from build123d import *

# Parameters (mm, degrees)
SKETCH_1_R          = 10
EXTRUDE_1_DEPTH     = 1
SKETCH_2_R          = 27.5
EXTRUDE_2_DEPTH     = 3.5
SKETCH_3_R          = 8.5
EXTRUDE_3_DEPTH     = 33
SKETCH_4_R          = 5
CUT_EXTRUDE_1_DEPTH = 20
EXTRUDE_START       = -37.5
EXTRUDE_4_DEPTH     = 37.5
SKETCH_9_R          = 1.5
CUT_EXTRUDE_4_DEPTH = 15
SKETCH_10_R         = 9.5
SKETCH_10_R_2       = 8.5
EXTRUDE_5_DEPTH     = 9.3
FILLET_2_R          = 8
CHAMFER_1_SIZE      = 0.5
CHAMFER_2_SIZE      = 0.5
SKETCH_12_R         = 1.5
CUT_EXTRUDE_6_DEPTH = 20
SKETCH_13_R         = 3.75
CUT_EXTRUDE_7_DEPTH = 44.732139257
FILLET_3_R          = 1
CHAMFER_3_SIZE      = 0.5
SKETCH_14_R         = 2.6
CUT_EXTRUDE_8_DEPTH = 10


with BuildPart() as part:
    # 草图1 → 凸台-拉伸1 (new body)
    with BuildSketch(Plane(origin=(0, 0, 0), x_dir=(1, 0, 0), z_dir=(0, 1, 0))):
        with Locations(Location((0, 0, 0), (0, 0, 270))):
            Circle(SKETCH_1_R)
    extrude(amount=EXTRUDE_1_DEPTH)

    # 草图2 → 凸台-拉伸2 (add)
    with BuildSketch(Plane(origin=(0, 1, 0), x_dir=(1, 0, 0), z_dir=(0, 1, 0))):
        with Locations(Location((0, 0, 0), (0, 0, 270))):
            Circle(SKETCH_2_R)
    extrude(amount=EXTRUDE_2_DEPTH)

    # 草图3 → 凸台-拉伸3 (add)
    with BuildSketch(Plane(origin=(0, 4.5, 0), x_dir=(1, 0, 0), z_dir=(0, 1, 0))):
        with Locations(Location((0, 0, 0), (0, 0, 270))):
            Circle(SKETCH_3_R)
    extrude(amount=EXTRUDE_3_DEPTH)

    # 草图4 → 切除-拉伸1 (cut)
    with BuildSketch(Plane(origin=(0, 37.5, 0), x_dir=(1, 0, 0), z_dir=(0, 1, 0))):
        with Locations(Location((0, 0, 0), (0, 0, 270))):
            Circle(SKETCH_4_R)
    extrude(amount=-CUT_EXTRUDE_1_DEPTH, mode=Mode.SUBTRACT)

    # 草图8 → 凸台-拉伸4 (add)
    with BuildSketch(Plane.XZ.offset(EXTRUDE_START)):
        with BuildLine():
            Line((4, 3), (4, -3))
            ThreePointArc((4, -3), (5, 0), (4, 3))
        make_face()
    extrude(amount=EXTRUDE_4_DEPTH)

    # 草图9 → 切除-拉伸4 (cut, symmetric)
    with BuildSketch(Plane.ZY.offset(-4)):
        with Locations((0, 28.5)):
            Circle(SKETCH_9_R)
    extrude(amount=CUT_EXTRUDE_4_DEPTH, both=True, mode=Mode.SUBTRACT)

    # 草图10 → 凸台-拉伸5 (add)
    with BuildSketch(Plane(origin=(0, 4.5, 0), x_dir=(1, 0, 0), z_dir=(0, 1, 0))):
        with Locations(Location((0, 0, 0), (0, 0, 270))):
            Circle(SKETCH_10_R)
        with Locations(Location((0, 0, 0), (0, 0, 270))):
            Circle(SKETCH_10_R_2, mode=Mode.SUBTRACT)
    extrude(amount=EXTRUDE_5_DEPTH)

    # 圆角2
    fillet_2_edges = [part.edges().sort_by_distance(p)[0] for p in [
        (0, 4.5, -9.5),
    ]]
    fillet(fillet_2_edges, radius=FILLET_2_R)

    # 倒角1
    chamfer_1_edges = [part.edges().sort_by_distance(p)[0] for p in [
        (0, 4.5, -27.5),
    ]]
    chamfer(chamfer_1_edges, length=CHAMFER_1_SIZE)

    # 倒角2
    chamfer_2_edges = [part.edges().sort_by_distance(p)[0] for p in [
        (0, 37.5, -8.5),
    ]]
    chamfer(chamfer_2_edges, length=CHAMFER_2_SIZE)

    # 草图12 → 切除-拉伸6 (cut)
    with BuildSketch(Plane(origin=(0, 37.5, 0), x_dir=(1, 0, 0), z_dir=(0, 1, 0))):
        with Locations((3, 3.5)):
            Circle(SKETCH_12_R)
        with Locations((3, -3.5)):
            Circle(SKETCH_12_R)
    extrude(amount=-CUT_EXTRUDE_6_DEPTH, mode=Mode.SUBTRACT)

    # 草图13 → 切除-拉伸7 (cut, through all)
    with BuildSketch(Plane(origin=(0, 17.5, 0), x_dir=(1, 0, 0), z_dir=(0, 1, 0))):
        with Locations(Location((0, 0, 0), (0, 0, 270))):
            Circle(SKETCH_13_R)
    extrude(amount=-CUT_EXTRUDE_7_DEPTH, mode=Mode.SUBTRACT)

    # 圆角3
    fillet_3_edges = [part.edges().sort_by_distance(p)[0] for p in [
        (1.973716593, 27.5, -4.593957206),
        (1.973716593, 27.5, 4.593957206),
    ]]
    fillet(fillet_3_edges, radius=FILLET_3_R)

    # 倒角3
    chamfer_3_edges = [part.edges().sort_by_distance(p)[0] for p in [
        (0, 1, -27.5),
    ]]
    chamfer(chamfer_3_edges, length=CHAMFER_3_SIZE)

    # 草图14 → 切除-拉伸8 (cut)
    with BuildSketch(Plane.XZ.offset(-1)):
        with Locations(Location((22.5, 0, 0), (0, 0, 270))):
            Circle(SKETCH_14_R)
        with Locations(Location((11.25, -19.485571585, 0), (0, 0, 270))):
            Circle(SKETCH_14_R)
        with Locations(Location((-11.25, -19.485571585, 0), (0, 0, 270))):
            Circle(SKETCH_14_R)
        with Locations(Location((-22.5, 0, 0), (0, 0, 270))):
            Circle(SKETCH_14_R)
        with Locations(Location((-11.25, 19.485571585, 0), (0, 0, 270))):
            Circle(SKETCH_14_R)
        with Locations(Location((11.25, 19.485571585, 0), (0, 0, 270))):
            Circle(SKETCH_14_R)
    extrude(amount=-CUT_EXTRUDE_8_DEPTH, mode=Mode.SUBTRACT)


solid = part.part
Part model, mm, in its own coordinate system. A direction names the side the tool comes from. Coordinates: 2 decimals unless noted, no trailing zeros. Write each loop counter-clockwise with the first axis right and the second up, starting at its lowest first coordinate (ties: lowest second). Pieces come first, ordered by that corner, then holes. Notation, with made-up numbers: M -35.5,-26 L -14.5,-26 A13 ccw -14.5,-15 Z; hole C 6.5,84.25 d4. An arc over 180 degrees is marked long. Return JSON: item names as keys, results as strings.
1. 3-axis set-ups, long thin cutter, end or side, ignore diameter. For faces 4 (the face through (0, 1, 12)), 5 (the face through (-12.246, 2.726, 17.084)), 6 (the face through (-5.78, 13.14, -7.54)): which of +Z, -Z, +X, -X, +Y, -Y reach the whole face in a straight line?
Determined:
{"face 4": "-Y", "face 5": "+Y, -Y", "face 6": "+Y"}
2. Probe L1, parallel to Y at x = -10.5, z = -16; L2, parallel to X at y = 23, z = -7; L3, parallel to X at y = 20, z = 4.5. List the from-to ranges inside material, lowest first.
Determined:
{"L1": "1 to 4.5", "L2": "-4.82 to 4.82", "L3": "-7.21 to -2.18, 4.12 to 7.21"}
3. Flat gauge pins, fed straight in: pin 1 Ø8.5 at (x, z) = (11.25, 19.49) entering from -Y; pin 2 Ø12 at (x, z) = (-14.5, -20.5) entering from +Y; pin 3 Ø1.4 at (y, z) = (29.5, -1) entering from -X. Where does each tip first touch, or does it go through?
Determined:
{"pin 1": "y = 1", "pin 2": "y = 4.5", "pin 3": "x = -8.49"}
4. Saw through at B-B, the plane y = 10.5. Write the cut outline in (x, z).
Determined:
{"outline": "C 0,0 d19.51; hole C 0,0 d7.5"}
5. Pull direction X, two halves, no side cores. Call faces 1 (the face through (-8.3, 25.24, -1.84)), 2 (the face through (6, 30, 0)), 3 (the face through (8.94, 2.73, 18.29)): pulls with the +X half, pulls with the -X half, needs draft (parallel to the pull), parting line crosses it, or undercut.
Determined:
{"face 1": "parting line crosses it", "face 2": "needs draft", "face 3": "undercut"}
6. Saw through at A-A, the plane z = 0. Count the separate pieces of the cut face and the enclosed holes in it, then the cut area to 3 significant figures.
Determined:
{"separate pieces": "6", "enclosed holes": "0", "area": "447 mm²"}
